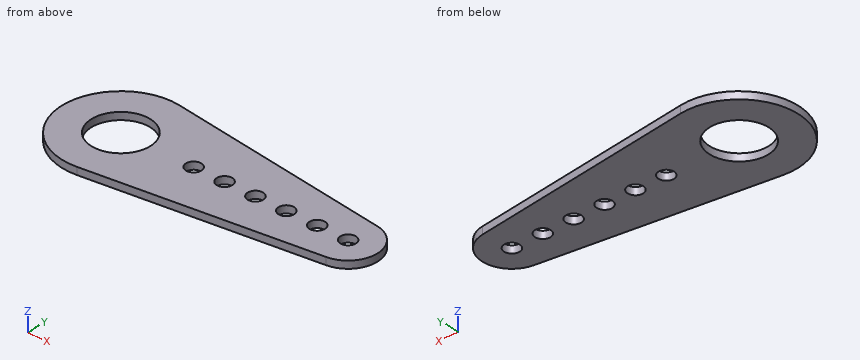
```python
from build123d import *

# Parameters (mm, degrees)
FLAT_SKETCH_R           = 25.4
FLAT_SKETCH_R_2         = 12.7
FLAT_SKETCH_R_3         = 3.3655
EXTRUDE_FACE_DEPTH      = 3.175
FLAT_SKETCH_4_R         = 3.3655
EXTRUDE_CUT_HOLES_DEPTH = 3.175


with BuildPart() as part:
    # Flat sketch → Extrude face (new body)
    # profile 1 of 13: a face of its own
    with BuildSketch(Plane.XY):
        Circle(FLAT_SKETCH_R)
        Circle(FLAT_SKETCH_R_2, mode=Mode.SUBTRACT)
    # profile 2 of 13: a face of its own
    with BuildSketch(Plane.XY):
        with BuildLine():
            Line((100.688205128, 12.595195436), (3.256410256, 25.190390871))
            ThreePointArc((3.256410256, 25.190390871), (19.077117451, 16.769722411), (25.4, 0))
            ThreePointArc((25.4, 0), (19.077117451, -16.769722411), (3.256410256, -25.190390871))
            Line((3.256410256, -25.190390871), (100.688205128, -12.595195436))
            ThreePointArc((100.688205128, -12.595195436), (91.936966729, -10.514389997), (86.759121462, -3.158858528))
            ThreePointArc((86.759121462, -3.158858528), (82.2325, 0), (86.759121462, 3.158858528))
            ThreePointArc((86.759121462, 3.158858528), (91.936966729, 10.514389997), (100.688205128, 12.595195436))
        make_face()
        with Locations((31.75, 0)):
            Circle(FLAT_SKETCH_R_3, mode=Mode.SUBTRACT)
        with Locations((45.212, 0)):
            Circle(FLAT_SKETCH_R_3, mode=Mode.SUBTRACT)
        with Locations((58.674, 0)):
            Circle(FLAT_SKETCH_R_3, mode=Mode.SUBTRACT)
        with Locations((72.136, 0)):
            Circle(FLAT_SKETCH_R_3, mode=Mode.SUBTRACT)
    # profile 3 of 13: a face of its own
    with BuildSketch(Plane.XY):
        with Locations((31.75, 0)):
            Circle(FLAT_SKETCH_R_3)
    # profile 4 of 13: a face of its own
    with BuildSketch(Plane.XY):
        with Locations((45.212, 0)):
            Circle(FLAT_SKETCH_R_3)
    # profile 5 of 13: a face of its own
    with BuildSketch(Plane.XY):
        with Locations((58.674, 0)):
            Circle(FLAT_SKETCH_R_3)
    # profile 6 of 13: a face of its own
    with BuildSketch(Plane.XY):
        with Locations((72.136, 0)):
            Circle(FLAT_SKETCH_R_3)
    # profile 7 of 13: a face of its own
    with BuildSketch(Plane.XY):
        with Locations((99.06, 0)):
            Circle(FLAT_SKETCH_R_2)
    # profile 8 of 13: a face of its own
    with BuildSketch(Plane.XY):
        with Locations((85.598, 0)):
            Circle(FLAT_SKETCH_R_3)
    # profile 9 of 13: a face of its own
    with BuildSketch(Plane.XY):
        with Locations((85.598, 0)):
            Circle(FLAT_SKETCH_R_3)
    # profile 10 of 13: a face of its own
    with BuildSketch(Plane.XY):
        with Locations((99.06, 0)):
            Circle(FLAT_SKETCH_R_2)
    # profile 11 of 13: a face of its own
    with BuildSketch(Plane.XY):
        with Locations((99.06, 0)):
            Circle(FLAT_SKETCH_R_2)
        with Locations((99.06, 0)):
            Circle(FLAT_SKETCH_R_3, mode=Mode.SUBTRACT)
    # profile 12 of 13: a face of its own
    with BuildSketch(Plane.XY):
        with Locations((85.598, 0)):
            Circle(FLAT_SKETCH_R_3)
    # profile 13 of 13: a face of its own
    with BuildSketch(Plane.XY):
        with Locations((99.06, 0)):
            Circle(FLAT_SKETCH_R_3)
    extrude(amount=EXTRUDE_FACE_DEPTH)

    # Flat sketch<4> → Extrude cut - holes (cut)
    with BuildSketch(Plane.XY):
        with Locations((99.06, 0)):
            Circle(FLAT_SKETCH_4_R)
        with Locations((85.598, 0)):
            Circle(FLAT_SKETCH_4_R)
        with Locations((72.136, 0)):
            Circle(FLAT_SKETCH_4_R)
        with Locations((58.674, 0)):
            Circle(FLAT_SKETCH_4_R)
        with Locations((45.212, 0)):
            Circle(FLAT_SKETCH_4_R)
        with Locations((31.75, 0)):
            Circle(FLAT_SKETCH_4_R)
    extrude(amount=EXTRUDE_CUT_HOLES_DEPTH, mode=Mode.SUBTRACT)


solid = part.part
```
Verification items for the finished model (mm, model axes). Round coordinates to 2 decimals unless told otherwise and drop trailing zeros. Write each loop counter-clockwise with the first axis right and the second up, starting at its lowest first coordinate (ties: lowest second). Pieces come first, ordered by that corner, then holes. Notation, with made-up numbers: (51.25, 53.25) - (69.25, 53.25) arc R24 ccw to (69.25, 85.25) - close; hole circle Ø8 at (71, 13.25). An arc over 180 degrees is marked (long way). Answer as a JSON object with one key per item and string values. Group by question number.
Q1. Thickness scan on line 1 (Y direction, x = 47, z = 1.4); line 2 (Y direction, x = 33, z = 1); line 3 (X direction, y = 5.5, z = 0.4). Record the ranges inside material, lowest first.
Q2. Section check D-D, the plane x = 64. Enter the section's corners in (y, z) (3 decimals), plus the area to 3 significant figures.
Q3. Section check C-C, the plane y = 6.5. Enter the section's corners in (x, z) (3 decimals), plus the area to 3 significant figures.
Q4. Section check B-B, the plane z = 0.85. Enter the section's corners in (x, y), plus the area to 3 significant figures.
Q5. Section check A-A, the plane x = 0. Enter the section's corners in (y, z) (3 decimals), plus the area to 3 significant figures.
Found:
{
 "1": {"line 1": "y = -19.54 to -2.85, 2.85 to 19.54", "line 2": "y = -21.35 to -3.12, 3.12 to 21.35", "line 3": "x = -24.8 to -11.45, 11.45 to 110.51"},
 "2": {"outline": "(-17.338, 0) - (17.338, 0) - (17.338, 3.175) - (-17.338, 3.175) - close", "area": "110 mm^2"},
 "3": {"outline": "(-24.554, 0) - (-10.911, 0) - (-10.911, 3.175) - (-24.554, 3.175) - close; (10.911, 0) - (109.971, 0) - (109.971, 3.175) - (10.911, 3.175) - close", "area": "358 mm^2"},
 "4": {"outline": "(3.26, -25.19) - (100.69, -12.6) arc R12.7 ccw to (100.69, 12.6) - (3.26, 25.19) arc R25.4 ccw (long way) to start; hole circle Ø25.4 at (0, 0); hole circle Ø6.73 at (31.75, 0); hole circle Ø6.73 at (45.21, 0); hole circle Ø6.73 at (58.67, 0); hole circle Ø6.73 at (72.14, 0); hole circle Ø6.73 at (85.6, 0); hole circle Ø6.73 at (99.06, 0)", "area": "4,350 mm^2"},
 "5": {"outline": "(-25.4, 0) - (-12.7, 0) - (-12.7, 3.175) - (-25.4, 3.175) - close; (12.7, 0) - (25.4, 0) - (25.4, 3.175) - (12.7, 3.175) - close", "area": "80.6 mm^2"}
}
